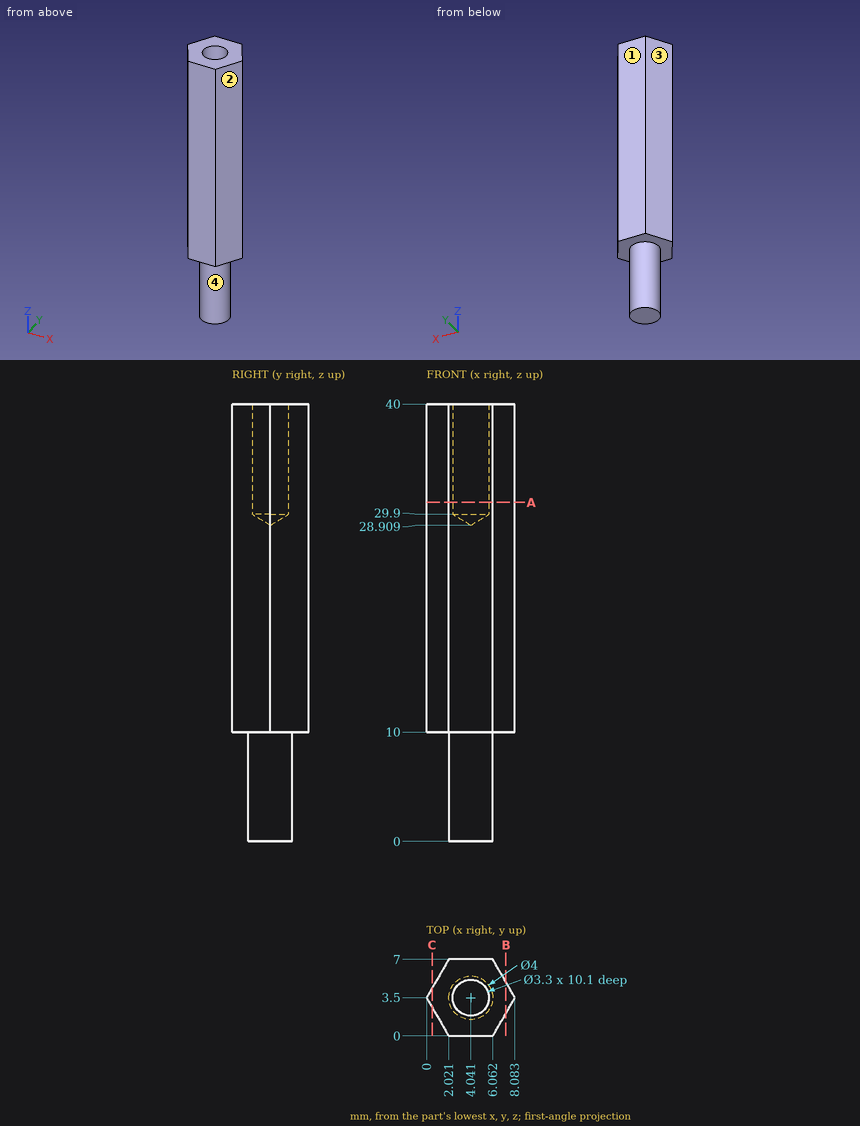
The figure shows three views and two pictorial views of one solid part (mm, origin at its lowest corner). Answer the questions. Give positions to 0.01 mm unless a question says otherwise; leave off trailing zeros. Loops run counter-clockwise (first coordinate to the right, second up) from the corner with the lowest first, then second, coordinate; pieces in that order, holes last. Notation, with made-up numbers: M 7.25,-25 L 36.25,-25 A25 ccw 36.25,-8 Z; hole C 20.5,34 d2. An arc over 180 degrees is marked long. Write each question's results on one line, items separated by ' | '.
1. Straight lines are drawn through the part: line 1 (Z direction, x = 6.5, y = 3.5); line 2 (X direction, y = 2.25, z = 21); line 3 (X direction, y = 5.25, z = 4.5) (1 decimal). For each, find the intervals that lie inside material, in ascending order. Write a range as [from, to].
Values:
line 1: z = [10, 40] | line 2: x = [0.72, 7.36] | line 3: x = [3.1, 5]
2. Section A-A on z = 31 is taken. Give the vertices of the cut face in (x, y).
Values:
outline: M 0,3.5 L 2.02,0 L 6.06,0 L 8.08,3.5 L 6.06,7 L 2.02,7 Z; hole C 4.04,3.5 d3.3
3. Section B-B on x = 7.25 is taken. Give the vertices of the cut face in (y, z).
Values:
outline: M 2.06,10 L 4.94,10 L 4.94,40 L 2.06,40 Z
4. The mould has two halves that part along X. Classify the marked faces 1, 2, 3 and 4: pulls with the +X half, pulls with the -X half, needs draft (parallel to the pull), parting line crosses it, or undercut.
Values:
face 1: needs draft | face 2: pulls with the +X half | face 3: pulls with the -X half | face 4: parting line crosses it
5. Given pin 1 (2 mm diameter, centred on x = 2, y = 4.5, fed in from -Z); pin 2 (4 mm diameter, centred on y = 0.5, z = 28, fed in from -X); pin 3 (1.5 mm diameter, centred on y = 6, z = 26, fed in from +X); pin 4 (2 mm diameter, centred on y = 4, z = 22, fed in from -X), each flat-ended and moving along its own axis, determine where each tip first touches the part or whether it passes through.
Values:
pin 1: stops at z = 0 | pin 2: stops at x = 0.58 | pin 3: stops at x = 7.07 | pin 4: stops at x = 0
6. Section C-C on x = 0.5 is taken. Give the vertices of the cut face in (y, z).
Values:
outline: M 2.63,10 L 4.37,10 L 4.37,40 L 2.63,40 Z
